Read the model definition and answer for the solid it produces. Units are mm, in the model's axes. A direction names the side the tool comes from. Coordinates: 2 decimals unless noted, no trailing zeros. Write each loop counter-clockwise with the first axis right and the second up, starting at its lowest first coordinate (ties: lowest second). Pieces come first, ordered by that corner, then holes. Notation, with made-up numbers: (-3.75, -23.75) -> (24.25, -23.75) arc R16 ccw to (24.25, 1.25) -> close; hole circle Ø3 at (36, 55). An arc over 180 degrees is marked (long way). Use CSV: the item, a comma, the result in double quotes.
from build123d import *

# Parameters (mm, degrees)
SKETCH1_R           = 6.5
SKETCH1_R_2         = 5
BOSS_EXTRUDE1_DEPTH = 5
SKETCH2_W           = 5
SKETCH2_H           = 5
BOSS_EXTRUDE2_DEPTH = 12.7
SKETCH3_R           = 5
CUT_EXTRUDE1_DEPTH  = 16.117539482


with BuildPart() as part:
    # Sketch1 → Boss-Extrude1 (new body)
    with BuildSketch(Plane(origin=(0, 0, 0), x_dir=(1, 0, 0), z_dir=(0, 1, 0))):
        with Locations(Location((0, 0, 0), (0, 0, 270))):
            Circle(SKETCH1_R)
        with Locations(Location((0, 0, 0), (0, 0, 270))):
            Circle(SKETCH1_R_2, mode=Mode.SUBTRACT)
    extrude(amount=BOSS_EXTRUDE1_DEPTH)

    # Sketch2 → Boss-Extrude2 (add, symmetric)
    with BuildSketch(Plane(origin=(0, 0, 0), x_dir=(0, -1, 0), z_dir=(-1, 0, 0))):
        with Locations((-2.5, 0)):
            Rectangle(SKETCH2_W, SKETCH2_H)
    extrude(amount=BOSS_EXTRUDE2_DEPTH, both=True)

    # Sketch3 → Cut-Extrude1 (cut, through all)
    with BuildSketch(Plane(origin=(0, 5, 0), x_dir=(1, 0, 0), z_dir=(0, 1, 0))):
        with Locations(Location((0, 0, 0), (0, 0, 270))):
            Circle(SKETCH3_R)
    extrude(amount=-CUT_EXTRUDE1_DEPTH, mode=Mode.SUBTRACT)


solid = part.part
1. A cutting plane is placed at A-A (x = 0). Give the vertices of the cut face in (y, z), and give its area (3 significant figures).
Solutions:
outline,"(0, -6.5) -> (5, -6.5) -> (5, -5) -> (0, -5) -> close; (0, 5) -> (5, 5) -> (5, 6.5) -> (0, 6.5) -> close"
area,"15.0 mm^2"
2. A cutting plane is placed at C-C (y = 1.75). Give the vertices of the cut face in (x, z).
Solutions:
outline,"(-12.7, -2.5) -> (-6, -2.5) arc R6.5 ccw to (6, -2.5) -> (12.7, -2.5) -> (12.7, 2.5) -> (6, 2.5) arc R6.5 ccw to (-6, 2.5) -> (-12.7, 2.5) -> close; hole circle Ø10 at (0, 0)"
3. A cutting plane is placed at D-D (x = 11). Give the vertices of the cut face in (y, z), and give its area (3 significant figures).
Solutions:
outline,"(0, -2.5) -> (5, -2.5) -> (5, 2.5) -> (0, 2.5) -> close"
area,"25.0 mm^2"
4. For a pull along Z with two mould halves and no side action, classify faces 1 (the cylindrical face through (0.1, 2.5, -6.5)), 2 (the flat face through (5, 0, 2)), 3 (the cylindrical face through (4.88, 2.46, 1.08)), 4 (the flat face through (9, 3, 2.5)) as pulls with the +Z half, pulls with the -Z half, needs draft (parallel to the pull), parting line crosses it, or undercut.
Solutions:
face 1,"pulls with the -Z half"
face 2,"needs draft"
face 3,"undercut"
face 4,"pulls with the +Z half"
5. Find the intervals of material crossed by line 1 along X through (y, z) = (3.7, 0); line 2 along Z through (x, y) = (-11.25, 2.9); line 3 along Z through (x, y) = (3, 4.45), in increasing order.
Solutions:
line 1,"x = -12.7 to -5, 5 to 12.7"
line 2,"z = -2.5 to 2.5"
line 3,"z = -5.77 to -4, 4 to 5.77"
6. A cutting plane is placed at B-B (z = 0). Give the vertices of the cut face in (x, y), and give its area (3 significant figures).
Solutions:
outline,"(-12.7, 0) -> (-5, 0) -> (-5, 5) -> (-12.7, 5) -> close; (5, 0) -> (12.7, 0) -> (12.7, 5) -> (5, 5) -> close"
area,"77.0 mm^2"
7. A tool of negligible diameter and unlimited length cuts with its end or side. For faces 5 (the flat face through (-9, 3, 2.5)), 6 (the flat face through (12.7, 3, 0)), 7 (the flat face through (9, 3, -2.5)), 8 (the flat face through (-9, 3, -2.5)), from which of +Z, -Z, +X, -X, +Y, -Y can it reach the whole face along a straight path? Write none if from no direction.
Solutions:
face 5,"+Z, -X, +Y, -Y"
face 6,"+Z, -Z, +X, +Y, -Y"
face 7,"-Z, +X, +Y, -Y"
face 8,"-Z, -X, +Y, -Y"
